Study the drawing (mm; zero at the part's minimum x, y, z) and answer. Coordinates: 2 decimals unless noted, no trailing zeros. Loops run counter-clockwise (first coordinate to the right, second up) from the corner with the lowest first, then second, coordinate; pieces in that order, holes last. Notation, with made-up numbers: (80.5, 58) -> (110.5, 58) arc R12 ccw to (110.5, 76) -> close; hole circle Ø1 at (49, 43.5). An arc over 180 degrees is marked (long way). Answer as a JSON object with one key per item and string values. Group by question number.
Q1. The part is cut by section C-C on x = 4.5. Write down the section's boundary in (y, z).
Q2. The part is cut by section A-A on z = 44.5. Write down the section's boundary in (x, y), and give its area (3 significant figures).
Q3. Straight lines are drawn through the part: line 1 along Y through (x, z) = (0.85, 44.5); line 2 along X through (y, z) = (73, 11.5); line 3 along X through (y, z) = (35, 48.5). For each, find the intervals that lie inside material, in ascending order. Write a range as [from, to].
Q4. Each of these flat-tipped pins is pushed along its axis until it touches: P1, Ø5, axis at x = 10.5, z = 68.5, coming from the -Y side; P2, Ø5, axis at x = 6, z = 61.5, coming from the +Y side; P3, Ø1.5, axis at x = 3, z = 41.5, coming from the -Y side. Where does it stop, or does it pass through?
Q5. The part is cut by section D-D on z = 67. Write down the section's boundary in (x, y), and give its area (3 significant figures).
Q6. Determine the mould class of the marked faces 1 and 2 for opening direction Z: released by +Z, released by -Z, zero draft, split by the parting line, or undercut.
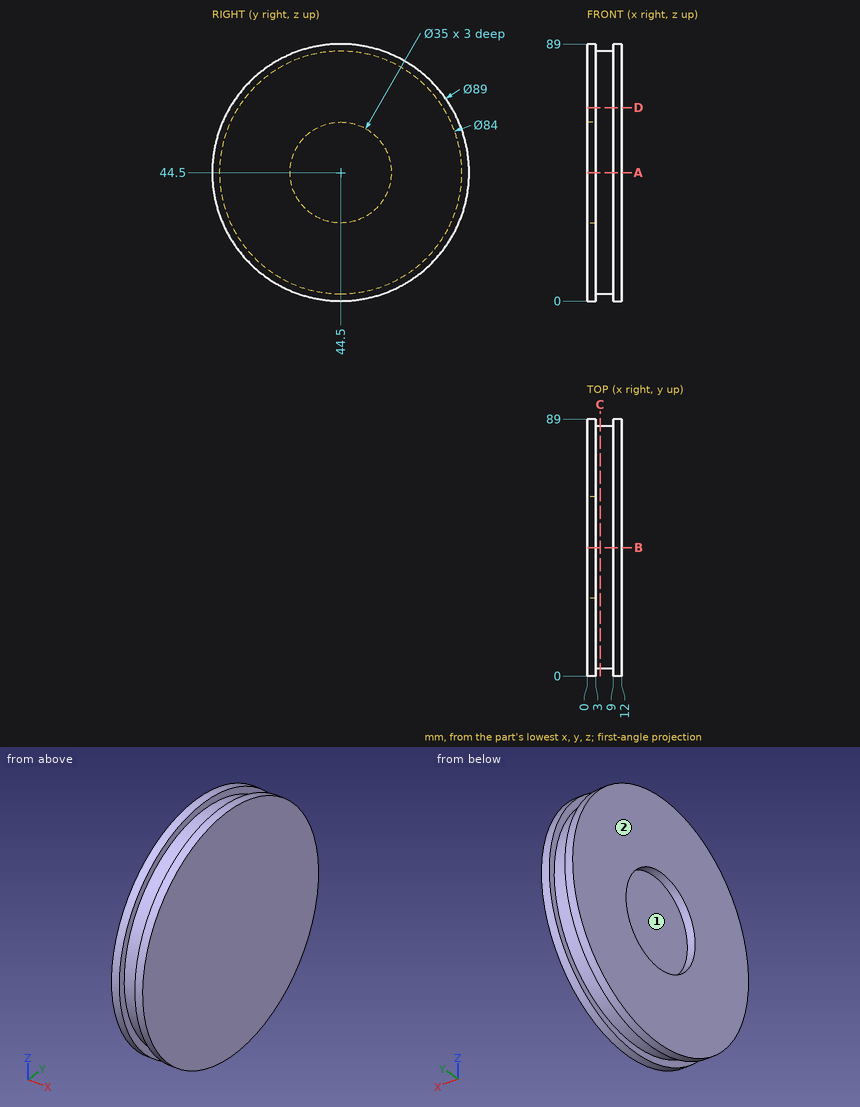
Final values:
{
 "1": {"outline": "circle Ø84 at (44.5, 44.5)"},
 "2": {"outline": "(0, 0) -> (3, 0) -> (3, 2.5) -> (9, 2.5) -> (9, 0) -> (12, 0) -> (12, 89) -> (9, 89) -> (9, 86.5) -> (3, 86.5) -> (3, 89) -> (0, 89) -> (0, 62) -> (3, 62) -> (3, 27) -> (0, 27) -> close", "area": "933 mm2"},
 "3": {"line 1": "y = [0, 27], [62, 89]", "line 2": "x = [0, 3], [9, 12]", "line 3": "x = [3, 12]"},
 "4": {"P1": "stops at y = 5.54", "P2": "stops at y = 83.92", "P3": "stops at y = 0.06"},
 "5": {"outline": "(0, 6.11) -> (3, 6.11) -> (3, 9.04) -> (9, 9.04) -> (9, 6.11) -> (12, 6.11) -> (12, 82.89) -> (9, 82.89) -> (9, 79.96) -> (3, 79.96) -> (3, 82.89) -> (0, 82.89) -> close", "area": "886 mm2"},
 "6": {"face 1": "undercut", "face 2": "zero draft"}
}
